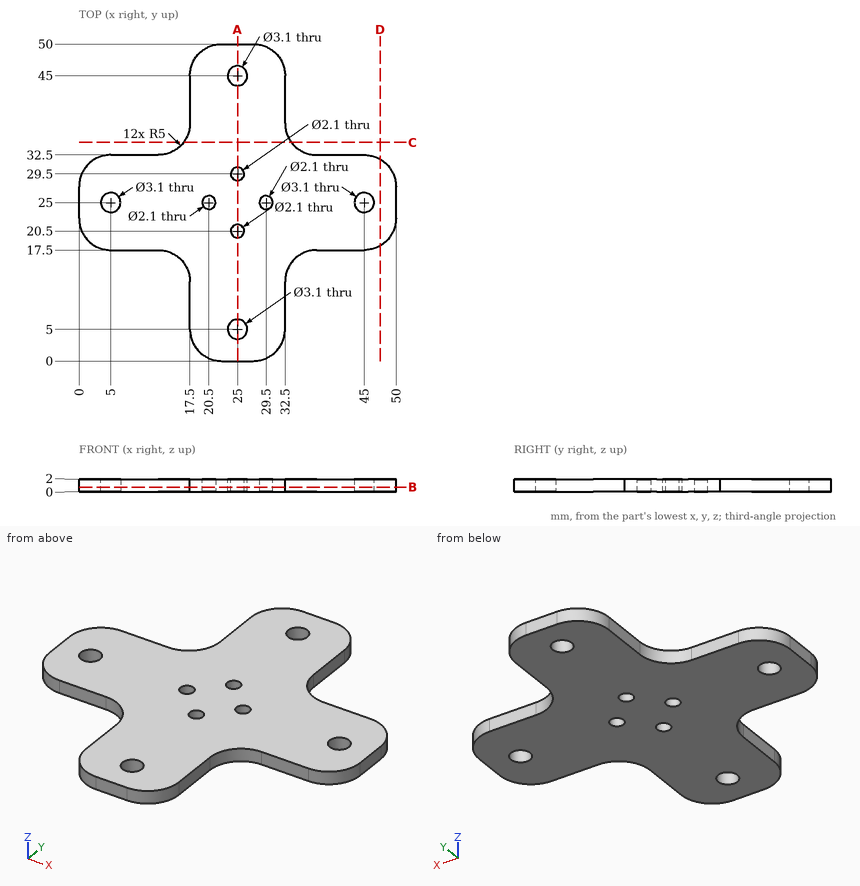
Drawing for the job (mm, zero at the part's lowest x, y, z). Round coordinates to 2 decimals unless told otherwise and drop trailing zeros. Write each loop counter-clockwise with the first axis right and the second up, starting at its lowest first coordinate (ties: lowest second). Pieces come first, ordered by that corner, then holes. Notation, with made-up numbers: (60, 6) - (105, 6) arc R16 cw to (105, 11) - close; hole circle Ø6 at (33.5, -38.75). An arc over 180 degrees is marked (long way). Return JSON: item names as keys, results as strings. Group by question number.
Item 1: Flat gauge pins, fed straight in: pin 1 Ø1.9 at (x, y) = (20.5, 25) entering from +Z; pin 2 Ø4 at (x, y) = (5, 25) entering from -Z; pin 3 Ø1 at (y, z) = (7.5, 1) entering from +X; pin 4 Ø0.6 at (x, z) = (40.5, 1) entering from -Y. Where does each tip first touch, or does it go through?
Item 2: Band-saw the part on B-B on z = 0.7. State how many separate pieces and enclosed holes the cut face has, plus the area to 3 significant figures.
Item 3: Band-saw the part on A-A on x = 25. List the corners of the cut face in (y, z), plus the area to 3 significant figures.
Item 4: Band-saw the part on D-D on x = 47.5. List the corners of the cut face in (y, z).
Item 5: Band-saw the part on C-C on y = 34.5. List the corners of the cut face in (x, z).
Item 6: Probe probe 1 along X at (y, z) = (45, 0.4); probe 2 along Y at (x, z) = (25.5, 1.4); probe 3 along Y at (x, z) = (40, 0.7). List the from-to ranges inside material, lowest first.
Resolved:
{
 "1": {"pin 1": "passes through", "pin 2": "stops at z = 0", "pin 3": "stops at x = 32.5", "pin 4": "stops at y = 17.5"},
 "2": {"separate pieces": "1", "enclosed holes": "8", "area": "1,210 mm²"},
 "3": {"outline": "(0, 0) - (3.45, 0) - (3.45, 2) - (0, 2) - close; (6.55, 0) - (19.45, 0) - (19.45, 2) - (6.55, 2) - close; (21.55, 0) - (28.45, 0) - (28.45, 2) - (21.55, 2) - close; (30.55, 0) - (43.45, 0) - (43.45, 2) - (30.55, 2) - close; (46.55, 0) - (50, 0) - (50, 2) - (46.55, 2) - close", "area": "79.2 mm²"},
 "4": {"outline": "(18.17, 0) - (31.83, 0) - (31.83, 2) - (18.17, 2) - close"},
 "5": {"outline": "(16.5, 0) - (33.5, 0) - (33.5, 2) - (16.5, 2) - close"},
 "6": {"probe 1": "x = 17.5 to 23.45, 26.55 to 32.5", "probe 2": "y = 0 to 3.53, 6.47 to 19.58, 21.42 to 28.58, 30.42 to 43.53, 46.47 to 50", "probe 3": "y = 17.5 to 32.5"}
}
